```python
from build123d import *

# Parameters (mm, degrees)
SKETCH1_W           = 90
SKETCH1_H           = 74
SKETCH1_W_2         = 86
SKETCH1_H_2         = 70
BOSS_EXTRUDE1_DEPTH = 25
BOSS_EXTRUDE2_START = 25
SKETCH1_3_W         = 10
SKETCH1_3_H         = 18
BOSS_EXTRUDE2_DEPTH = 25
SKETCH2_W           = 86
SKETCH2_H           = 70
BOSS_EXTRUDE3_DEPTH = 2
SKETCH3_W           = 3.2
SKETCH3_H           = 4.098780306
CUT_EXTRUDE1_DEPTH  = 2
SKETCH3_4_R         = 4.1
SKETCH3_4_R_2       = 2.6
BOSS_EXTRUDE4_DEPTH = 7.5
SKETCH4_R           = 6
CUT_EXTRUDE2_DEPTH  = 2
BOSS_EXTRUDE5_START = -2
BOSS_EXTRUDE5_DEPTH = 2
BOSS_EXTRUDE6_START = -2
SKETCH4_4_W         = 16.2
SKETCH4_4_H         = 2
SKETCH4_4_W_2       = 2
SKETCH4_4_H_2       = 10
BOSS_EXTRUDE6_DEPTH = 9
SKETCH6_R           = 1.5
BOSS_EXTRUDE7_DEPTH = 5
SKETCH7_R           = 2.5
BOSS_EXTRUDE8_DEPTH = 3
CUT_EXTRUDE3_DEPTH  = 106.019045892


with BuildPart() as part:
    # Sketch1 → Boss-Extrude1 (new, symmetric)
    with BuildSketch(Plane.XY):
        Rectangle(SKETCH1_W, SKETCH1_H)
        Rectangle(SKETCH1_W_2, SKETCH1_H_2, mode=Mode.SUBTRACT)
    extrude(amount=BOSS_EXTRUDE1_DEPTH, both=True)

    # Sketch1<3> → Boss-Extrude2 (add)
    with BuildSketch(Plane.XY.offset(BOSS_EXTRUDE2_START)):
        with Locations((-20, -46)):
            Rectangle(SKETCH1_3_W, SKETCH1_3_H)
        with Locations((20, -46)):
            Rectangle(SKETCH1_3_W, SKETCH1_3_H)
    extrude(amount=-BOSS_EXTRUDE2_DEPTH)

    # Sketch2 → Boss-Extrude3 (add)
    with BuildSketch(Plane(origin=(0, 0, -25), x_dir=(-1, 0, 0), z_dir=(0, 0, -1))):
        Rectangle(SKETCH2_W, SKETCH2_H)
    extrude(amount=-BOSS_EXTRUDE3_DEPTH)

    # Sketch3 → Cut-Extrude1 (cut)
    with BuildSketch(Plane(origin=(0, 37, 0), x_dir=(1, 0, 0), z_dir=(0, 1, 0))):
        with BuildLine():
            Line((-1.6, 2.049390153), (1.6, 2.049390153))
            ThreePointArc((1.6, 2.049390153), (0, 2.6), (-1.6, 2.049390153))
        make_face()
        Rectangle(SKETCH3_W, SKETCH3_H)
        with BuildLine():
            ThreePointArc((-1.6, -2.049390153), (0, -2.6), (1.6, -2.049390153))
            Line((1.6, -2.049390153), (-1.6, -2.049390153))
        make_face()
    extrude(amount=-CUT_EXTRUDE1_DEPTH, mode=Mode.SUBTRACT)

    # Sketch3<4> → Boss-Extrude4 (add)
    # profile 1 of 3: a face of its own
    with BuildSketch(Plane(origin=(0, 37, 0), x_dir=(1, 0, 0), z_dir=(0, 1, 0))):
        with Locations(Location((0, 0, 0), (0, 0, 270))):
            Circle(SKETCH3_4_R)
        Circle(SKETCH3_4_R_2, mode=Mode.SUBTRACT)
    # profile 2 of 3: a face of its own
    with BuildSketch(Plane(origin=(0, 37, 0), x_dir=(1, 0, 0), z_dir=(0, 1, 0))):
        with BuildLine():
            Line((1.6, 2.049390153), (1.6, -2.049390153))
            ThreePointArc((1.6, -2.049390153), (2.336664289, -1.140175425), (2.6, 0))
            ThreePointArc((2.6, 0), (2.336664289, 1.140175425), (1.6, 2.049390153))
        make_face()
    # profile 3 of 3: a face of its own
    with BuildSketch(Plane(origin=(0, 37, 0), x_dir=(1, 0, 0), z_dir=(0, 1, 0))):
        with BuildLine():
            ThreePointArc((-1.6, 2.049390153), (-2.6, 0), (-1.6, -2.049390153))
            Line((-1.6, -2.049390153), (-1.6, 2.049390153))
        make_face()
    extrude(amount=-BOSS_EXTRUDE4_DEPTH)

    # Sketch4 → Cut-Extrude2 (cut)
    with BuildSketch(Plane(origin=(45, 0, 0), x_dir=(0, 0, -1), z_dir=(1, 0, 0))):
        Circle(SKETCH4_R)
        with BuildLine():
            Line((3.5, -8.831760866), (3.5, -4.873397172))
            ThreePointArc((3.5, -4.873397172), (0, -6), (-3.5, -4.873397172))
            Line((-3.5, -4.873397172), (-3.5, -8.831760866))
            ThreePointArc((-3.5, -8.831760866), (0, -9.5), (3.5, -8.831760866))
        make_face()
    extrude(amount=-CUT_EXTRUDE2_DEPTH, mode=Mode.SUBTRACT)

    # Sketch4<3> → Boss-Extrude5 (add)
    with BuildSketch(Plane(origin=(45, 0, 0), x_dir=(0, 0, -1), z_dir=(1, 0, 0)).offset(BOSS_EXTRUDE5_START)):
        with BuildLine():
            ThreePointArc((6, 0), (5.338539126, -2.738612788), (3.5, -4.873397172))
            Line((3.5, -4.873397172), (3.5, -8.831760866))
            ThreePointArc((3.5, -8.831760866), (7.858116823, -5.338539126), (9.5, 0))
            ThreePointArc((9.5, 0), (-5.338539126, 7.858116823), (-3.5, -8.831760866))
            Line((-3.5, -8.831760866), (-3.5, -4.873397172))
            ThreePointArc((-3.5, -4.873397172), (-2.738612788, 5.338539126), (6, 0))
        make_face()
    extrude(amount=-BOSS_EXTRUDE5_DEPTH)

    # Sketch4<4> → Boss-Extrude6 (add)
    with BuildSketch(Plane(origin=(45, 0, 0), x_dir=(0, 0, -1), z_dir=(1, 0, 0)).offset(BOSS_EXTRUDE6_START)):
        with Locations((0, 11.5)):
            Rectangle(SKETCH4_4_W, SKETCH4_4_H)
        with Locations((-7.1, -17)):
            Rectangle(SKETCH4_4_W_2, SKETCH4_4_H_2)
        with Locations((0, -23)):
            Rectangle(SKETCH4_4_W, SKETCH4_4_H)
        with Locations((7.1, -17)):
            Rectangle(SKETCH4_4_W_2, SKETCH4_4_H_2)
        with Locations((-7.1, 9.5)):
            Rectangle(SKETCH4_4_W_2, SKETCH4_4_H)
        with Locations((7.1, 9.5)):
            Rectangle(SKETCH4_4_W_2, SKETCH4_4_H)
    extrude(amount=-BOSS_EXTRUDE6_DEPTH)

    # Sketch6 → Boss-Extrude7 (add)
    with BuildSketch(Plane.XY.offset(-23)):
        with Locations((32.25, 3.5)):
            Circle(SKETCH6_R)
        with Locations((-18.75, 19.25)):
            Circle(SKETCH6_R)
        with Locations((-19.75, -29.25)):
            Circle(SKETCH6_R)
        with Locations((32.25, -24)):
            Circle(SKETCH6_R)
    extrude(amount=BOSS_EXTRUDE7_DEPTH)

    # Sketch7 → Boss-Extrude8 (add)
    with BuildSketch(Plane.ZY.offset(45)):
        Circle(SKETCH7_R)
    extrude(amount=BOSS_EXTRUDE8_DEPTH)

    # Sketch8 → Cut-Extrude3 (cut, through all)
    with BuildSketch(Plane.XZ.offset(-35)):
        with BuildLine():
            ThreePointArc((11.490666647, -9.641814145), (0, -15), (-11.490666647, -9.641814145))
            Line((-11.490666647, -9.641814145), (-15.320888862, -12.855752194))
            ThreePointArc((-15.320888862, -12.855752194), (0, -20), (15.320888862, -12.855752194))
            Line((15.320888862, -12.855752194), (11.490666647, -9.641814145))
        make_face()
        with BuildLine():
            Line((-15.320888862, -12.855752194), (-11.490666647, -9.641814145))
            ThreePointArc((-11.490666647, -9.641814145), (-15.012746779, -9.333672062), (-15.320888862, -12.855752194))
        make_face()
        with BuildLine():
            ThreePointArc((15.320888862, -12.855752194), (15.012746779, -9.333672062), (11.490666647, -9.641814145))
            Line((11.490666647, -9.641814145), (15.320888862, -12.855752194))
        make_face()
    extrude(amount=-CUT_EXTRUDE3_DEPTH, mode=Mode.SUBTRACT)


solid = part.part
```
Read the model definition and answer for the solid it produces. Units are mm, in the model's axes. A direction names the side the tool comes from. Coordinates: 2 decimals unless noted, no trailing zeros. Write each loop counter-clockwise with the first axis right and the second up, starting at its lowest first coordinate (ties: lowest second). Pieces come first, ordered by that corner, then holes. Notation, with made-up numbers: (-25.5, 66) - (13.5, 66) arc R26 cw to (13.5, 82) - close; hole circle Ø7 at (4, 44.5). An arc over 180 degrees is marked (long way). Answer as a JSON object with one key per item and string values. Group by question number.
1. A cutting plane is placed at B-B (y = -33). Determine the outline of the cut face in (x, z), plus the area to 3 significant figures.
2. The mould has two halves that part along Z. Classify faces 4 (the cylindrical face through (0, 33.3, 2.6)), 5 (the flat face through (20, -46, 0)), 6 (the flat face through (-20, -55, 13)): +Z half, -Z half, draft (parallel to the pull), parting line (faces both ways), or undercut.
3. Consider L1, parallel to Y at x = 41.75, z = 0; L2, parallel to Z at x = 41, y = 10; L3, parallel to X at y = 5.5, z = 3.5. Determine where each line is inside the solid, lowest interval first. Write a range as [from, to].
4. Which of the six approach directions +Z, -Z, +X, -X, +Y, -Y give full straight-line access (tool end or side, diameter ignored) to faces 1 (the flat face through (25, -46, 13)), 2 (the flat face through (39, 10, -8.1)), 3 (the cylindrical face through (0, 36, -20))?
5. A cutting plane is placed at C-C (x = -29). Determine the outline of the cut face in (y, z).
6. A cutting plane is placed at A-A (x = 36). Determine the outline of the cut face in (y, z), plus the area to 3 significant figures.
7. A cutting plane is placed at D-D (y = 19.25). Determine the outline of the cut face in (x, z).
8. Each of these flat-tipped pins is pushed along its axis until it touches: P1, Ø0.6, axis at x = 37, y = 9.5, coming from the +Z side; P2, Ø4, axis at x = 17, z = -14.5, coming from the -Y side; P3, Ø4, axis at x = -10.5, y = 26.5, coming from the +Z side; P4, Ø2, axis at x = 42.5, y = -7, coming from the +Z side. Where does it stop, or does it pass through?
Worked out:
{
 "1": {"outline": "(-45, -25) - (45, -25) - (45, 25) - (43, 25) - (43, -23) - (-43, -23) - (-43, 25) - (-45, 25) - close", "area": "372 mm²"},
 "2": {"face 4": "undercut", "face 5": "-Z half", "face 6": "draft"},
 "3": {"L1": "y = [-37, -35], [-24, -22], [6, 9.5], [10.5, 12.5], [35, 37]", "L2": "z = [-25, -23], [-8.1, -6.1], [6.1, 8.1]", "L3": "x = [-45, -43], [41, 45]"},
 "4": {"face 1": "+Z, -Z, +X, -Y", "face 2": "none", "face 3": "+Y"},
 "5": {"outline": "(-37, -25) - (37, -25) - (37, 25) - (35, 25) - (35, -23) - (-35, -23) - (-35, 25) - (-37, 25) - close"},
 "6": {"outline": "(-37, -25) - (37, -25) - (37, 25) - (35, 25) - (35, -23) - (-35, -23) - (-35, 25) - (-37, 25) - close; (-24, -8.1) - (-12, -8.1) - (-12, -6.1) - (-22, -6.1) - (-22, 6.1) - (-12, 6.1) - (-12, 8.1) - (-24, 8.1) - close; (8.5, -8.1) - (12.5, -8.1) - (12.5, 8.1) - (8.5, 8.1) - (8.5, 6.1) - (10.5, 6.1) - (10.5, -6.1) - (8.5, -6.1) - close", "area": "453 mm²"},
 "7": {"outline": "(-45, -25) - (45, -25) - (45, 25) - (43, 25) - (43, -23) - (-17.25, -23) - (-17.25, -18) - (-20.25, -18) - (-20.25, -23) - (-43, -23) - (-43, 25) - (-45, 25) - close"},
 "8": {"P1": "stops at z = 8.1", "P2": "stops at y = -37", "P3": "stops at z = -23", "P4": "stops at z = 25"}
}
